For this review, take the finished solid that the model builds, in its own axes (mm). A direction names the side the tool comes from. Round coordinates to 2 decimals unless told otherwise and drop trailing zeros. Loops run counter-clockwise (first coordinate to the right, second up) from the corner with the lowest first, then second, coordinate; pieces in that order, holes last.
```python
from build123d import *

# Parameters (mm, degrees)
SKETCH1_R           = 1.65
BOSS_EXTRUDE1_DEPTH = 3
SKETCH1_3_R         = 1.65
CUT_EXTRUDE1_DEPTH  = 2.1
FILLET3_R           = 2
SKETCH2_W           = 29
SKETCH2_H           = 2
BOSS_EXTRUDE2_DEPTH = 3
SKETCH2_3_W         = 29
SKETCH2_3_H         = 3
BOSS_EXTRUDE3_DEPTH = 13
CUT_EXTRUDE2_DEPTH  = 33.975900291
CUT_EXTRUDE3_DEPTH  = 2.1


with BuildPart() as part:
    # Sketch1 → Boss-Extrude1 (new body)
    with BuildSketch(Plane.XY):
        with BuildLine():
            Line((0, 0), (29, 0))
            Line((29, 0), (29, 10.1))
            Line((29, 10.1), (22, 10.1))
            Line((22, 10.1), (22, 7))
            ThreePointArc((22, 7), (21.853553391, 6.646446609), (21.5, 6.5))
            Line((21.5, 6.5), (7.5, 6.5))
            ThreePointArc((7.5, 6.5), (7.146446609, 6.646446609), (7, 7))
            Line((7, 7), (7, 10.1))
            Line((7, 10.1), (0, 10.1))
            Line((0, 10.1), (0, 0))
        make_face()
        with Locations((4.75, 6)):
            Circle(SKETCH1_R, mode=Mode.SUBTRACT)
        with Locations((24.25, 6)):
            Circle(SKETCH1_R, mode=Mode.SUBTRACT)
    extrude(amount=BOSS_EXTRUDE1_DEPTH)

    # Sketch1_3 → Cut-Extrude1 (cut)
    # profile 1 of 2: a face of its own
    with BuildSketch(Plane.XY):
        with BuildLine():
            Line((2.960214166, 9.1), (1.170428331, 6))
            Line((1.170428331, 6), (2.960214166, 2.9))
            Line((2.960214166, 2.9), (6.539785834, 2.9))
            Line((6.539785834, 2.9), (8.329571669, 6))
            Line((8.329571669, 6), (8.040896534, 6.5))
            Line((8.040896534, 6.5), (7.5, 6.5))
            ThreePointArc((7.5, 6.5), (7.146446609, 6.646446609), (7, 7))
            Line((7, 7), (7, 9.1))
            Line((7, 9.1), (2.960214166, 9.1))
        make_face()
        with Locations((4.75, 6)):
            Circle(SKETCH1_3_R, mode=Mode.SUBTRACT)
    # profile 2 of 2: a face of its own
    with BuildSketch(Plane.XY):
        with BuildLine():
            Line((27.829571669, 6), (26.039785834, 9.1))
            Line((26.039785834, 9.1), (22, 9.1))
            Line((22, 9.1), (22, 7))
            ThreePointArc((22, 7), (21.853553391, 6.646446609), (21.5, 6.5))
            Line((21.5, 6.5), (20.959103466, 6.5))
            Line((20.959103466, 6.5), (20.670428331, 6))
            Line((20.670428331, 6), (22.460214166, 2.9))
            Line((22.460214166, 2.9), (26.039785834, 2.9))
            Line((26.039785834, 2.9), (27.829571669, 6))
        make_face()
        with Locations((24.25, 6)):
            Circle(SKETCH1_3_R, mode=Mode.SUBTRACT)
    extrude(amount=CUT_EXTRUDE1_DEPTH, mode=Mode.SUBTRACT)

    # Fillet3
    fillet3_edges = [part.edges().sort_by_distance(p)[0] for p in [
        (7, 10.1, 1.5),
        (22, 10.1, 1.5),
    ]]
    fillet(fillet3_edges, radius=FILLET3_R)

    # Sketch2 → Boss-Extrude2 (add)
    with BuildSketch(Plane.XY.offset(3)):
        with Locations((14.5, -1)):
            Rectangle(SKETCH2_W, SKETCH2_H)
    extrude(amount=-BOSS_EXTRUDE2_DEPTH)

    # Sketch2_3 → Boss-Extrude3 (add)
    with BuildSketch(Plane.XY.offset(3)):
        with Locations((14.5, -3.5)):
            Rectangle(SKETCH2_3_W, SKETCH2_3_H)
    extrude(amount=-BOSS_EXTRUDE3_DEPTH)

    # Sketch3 → Cut-Extrude2 (cut, through all)
    with BuildSketch(Plane(origin=(0, -2, 0), x_dir=(1, 0, 0), z_dir=(0, 1, 0))):
        with BuildLine():
            ThreePointArc((20.15, 5), (21.75, 3.4), (23.35, 5))
            Line((23.35, 5), (21.75, 5))
            Line((21.75, 5), (20.15, 5))
        make_face()
        with BuildLine():
            Line((21.75, 5), (23.35, 5))
            ThreePointArc((23.35, 5), (21.75, 6.6), (20.15, 5))
            Line((20.15, 5), (21.75, 5))
        make_face()
        with BuildLine():
            ThreePointArc((5.65, 5), (7.25, 3.4), (8.85, 5))
            Line((8.85, 5), (7.25, 5))
            Line((7.25, 5), (5.65, 5))
        make_face()
        with BuildLine():
            Line((7.25, 5), (8.85, 5))
            ThreePointArc((8.85, 5), (7.25, 6.6), (5.65, 5))
            Line((5.65, 5), (7.25, 5))
        make_face()
    extrude(amount=-CUT_EXTRUDE2_DEPTH, mode=Mode.SUBTRACT)

    # Sketch3_3 → Cut-Extrude3 (cut)
    with BuildSketch(Plane(origin=(0, -2, 0), x_dir=(1, 0, 0), z_dir=(0, 1, 0))):
        with BuildLine():
            Line((23.539785834, 1.9), (25.329571669, 5))
            Line((25.329571669, 5), (23.35, 5))
            ThreePointArc((23.35, 5), (21.75, 3.4), (20.15, 5))
            Line((20.15, 5), (18.170428331, 5))
            Line((18.170428331, 5), (19.960214166, 1.9))
            Line((19.960214166, 1.9), (23.539785834, 1.9))
        make_face()
        with BuildLine():
            Line((23.35, 5), (25.329571669, 5))
            Line((25.329571669, 5), (23.539785834, 8.1))
            Line((23.539785834, 8.1), (19.960214166, 8.1))
            Line((19.960214166, 8.1), (18.170428331, 5))
            Line((18.170428331, 5), (20.15, 5))
            ThreePointArc((20.15, 5), (21.75, 6.6), (23.35, 5))
        make_face()
        with BuildLine():
            Line((9.039785834, 1.9), (10.829571669, 5))
            Line((10.829571669, 5), (8.85, 5))
            ThreePointArc((8.85, 5), (7.25, 3.4), (5.65, 5))
            Line((5.65, 5), (3.670428331, 5))
            Line((3.670428331, 5), (5.460214166, 1.9))
            Line((5.460214166, 1.9), (9.039785834, 1.9))
        make_face()
        with BuildLine():
            Line((8.85, 5), (10.829571669, 5))
            Line((10.829571669, 5), (9.039785834, 8.1))
            Line((9.039785834, 8.1), (5.460214166, 8.1))
            Line((5.460214166, 8.1), (3.670428331, 5))
            Line((3.670428331, 5), (5.65, 5))
            ThreePointArc((5.65, 5), (7.25, 6.6), (8.85, 5))
        make_face()
    extrude(amount=-CUT_EXTRUDE3_DEPTH, mode=Mode.SUBTRACT)


solid = part.part
```
(1) Add section A-A (x = 4). Give the boundary of the cut face in (y, z).
(2) The part is to be moulded in two halves that separate along X. For faces 5 (the flat face through (29, -1, 1)), 6 (the flat face through (14, -5, -3)), 7 (the flat face through (26, 5, 2.1)), say which applies: pulls with the +X half, pulls with the -X half, needs draft (parallel to the pull), parting line crosses it, or undercut.
(3) Add section B-B (z = 1). Give the boundary of the cut face in (x, y), plus the area to 3 significant figures.
(4) Insertion check: pin 1 Ø1 at (y, z) = (7.5, 2.5) entering from -X; pin 2 Ø5 at (x, z) = (22, -4.5) entering from +Y; pin 3 Ø6 at (x, y) = (17.5, 4) entering from -Z; pin 4 Ø1.9 at (x, y) = (5.5, 6.5) entering from -Z. Each pin has a flat end and moves straight along its axis. Give the tip position at first contact, or say it passes through.
(5) For L1, parallel to X at y = -4.4, z = -5; L2, parallel to X at y = -2.5, z = -2.5; L3, parallel to Y at x = 24, z = 1, list the stretches that pass through material, from the lowest coordinate up.
(6) For faces 1 (the flat face through (3, 5, 2.1)), 2 (the flat face through (9.947, -3.035, -6.528)), 3 (the flat face through (14, -2, -5)), 4 (the flat face through (22, 7.6, 2.5)), list the 3-axis set-ups (+Z, -Z, +X, -X, +Y, -Y) from which the entire face can be reached by the end or side of a thin tool; tool diameter is ignored.
(7) Add section D-D (z = -4). Give the boundary of the cut face in (x, y), plus the area to 3 significant figures.
(8) Add section C-C (x = 17.5). Give the boundary of the cut face in (y, z).
Outcome:
1. outline: (-5, -10) - (-2, -10) - (-2, -5.57) - (-4.1, -5.57) - (-4.1, -4.43) - (-2, -4.43) - (-2, 0) - (2.9, 0) - (2.9, 2.1) - (4.53, 2.1) - (4.53, 3) - (-5, 3) - close; (7.47, 2.1) - (9.1, 2.1) - (9.1, 0) - (10.1, 0) - (10.1, 3) - (7.47, 3) - close
2. face 5: pulls with the +X half
2. face 6: needs draft
2. face 7: undercut
3. outline: (0, -5) - (29, -5) - (29, 10.1) - (24, 10.1) arc R2 ccw to (22.27, 9.1) - (26.04, 9.1) - (27.83, 6) - (26.04, 2.9) - (22.46, 2.9) - (20.67, 6) - (20.96, 6.5) - (8.04, 6.5) - (8.33, 6) - (6.54, 2.9) - (2.96, 2.9) - (1.17, 6) - (2.96, 9.1) - (6.73, 9.1) arc R2 ccw to (5, 10.1) - (0, 10.1) - close
3. area: 317 mm2
4. pin 1: stops at x = 0
4. pin 2: stops at y = -4.1
4. pin 3: stops at z = 0
4. pin 4: stops at z = 2.1
5. L1: x = 0 to 5.65, 8.85 to 20.15, 23.35 to 29
5. L2: x = 0 to 5.11, 9.39 to 19.61, 23.89 to 29
5. L3: y = -5 to 2.9, 9.1 to 10.1
6. face 1: -Z
6. face 2: +Y
6. face 3: -Z, +X, -X, +Y
6. face 4: +Z, -Z, +Y
7. outline: (0, -5) - (6, -5) - (6, -4.1) - (4.25, -4.1) - (4.25, -2) - (0, -2) - close; (8.5, -5) - (20.5, -5) - (20.5, -4.1) - (18.75, -4.1) - (18.75, -2) - (10.25, -2) - (10.25, -4.1) - (8.5, -4.1) - close; (23, -5) - (29, -5) - (29, -2) - (24.75, -2) - (24.75, -4.1) - (23, -4.1) - close
7. area: 57.3 mm2
8. outline: (-5, -10) - (-2, -10) - (-2, 0) - (6.5, 0) - (6.5, 3) - (-5, 3) - close
